Input: part model. Units: mm. Frame: model coordinates. Round coordinates to 2 decimals unless told otherwise and drop trailing zeros. Write each loop counter-clockwise with the first axis right and the second up, starting at its lowest first coordinate (ties: lowest second). Pieces come first, ordered by that corner, then holes. Notation, with made-up numbers: (47, -37) -> (51, -37) arc R32 cw to (51, -3) -> close; hole circle Ø2 at (21.5, 70.25). An arc over 180 degrees is marked (long way). Use CSV: the item, a comma, the result in double quotes.
Autodesk Inventor part; units mm, degrees
ref_plane "YZ Plane" through (0, 0, 0) normal (1, 0, 0) x (0, 1, 0)
ref_plane "XZ Plane" through (0, 0, 0) normal (0, 1, 0) x (-1, 0, 0)
ref_plane "XY Plane" through (0, 0, 0) normal (0, 0, 1) x (1, 0, 0)
sketch "Sketch1" plane through (0, 0, 0) normal (0, 1, 0) x (-1, 0, 0)
  line L0 (16.1925, 35.7868) -> (-9.2075, 35.7868)
  line L1 (-9.2075, 35.7868) -> (-9.2075, 10.3868)
  line L2 (-9.2075, 10.3868) -> (16.1925, 10.3868)
  line L3 (16.1925, 10.3868) -> (16.1925, 35.7868)
  point P0 (0, 0)
  dimension "d0" = 25.4
  dimension "d1" = 25.4
extrude "Extrusion1" add sketch "Sketch1" along normal blind 368.3
sketch "Sketch2" plane through (0, 368.3, 0) normal (0, 1, 0) x (1, 0, 0)
  line L0 (-9.8425, -16.7368) -> (2.8575, -16.7368)
  line L1 (2.8575, -16.7368) -> (2.8575, -1.003)
  line L2 (2.8575, -1.003) -> (-9.8425, -1.003)
  line L3 (-9.8425, -1.003) -> (-9.8425, -16.7368)
  line L4 (9.2075, -35.7868) -> (9.2075, -10.3868)
  line L5 (-16.1925, -10.3868) -> (-16.1925, -35.7868)
  line L6 (9.2075, -10.3868) -> (-16.1925, -10.3868)
  point P0 (0, 0)
  dimension "d4" = 6.35
  dimension "d5" = 6.35
  dimension "d6" = 6.35
extrude "Extrusion2" cut sketch "Sketch2" against normal blind 508
sketch "Sketch4" plane through (0, 368.3, 0) normal (0, 1, 0) x (1, 0, 0)
  line L0 (-9.8425, -29.4368) -> (2.8575, -29.4368)
  line L1 (2.8575, -29.4368) -> (2.8575, -45.8861)
  line L2 (2.8575, -45.8861) -> (-9.8425, -45.8861)
  line L3 (-9.8425, -45.8861) -> (-9.8425, -29.4368)
  line L4 (-16.1925, -10.3868) -> (-16.1925, -35.7868)
  line L5 (9.2075, -35.7868) -> (9.2075, -10.3868)
  line L6 (-16.1925, -35.7868) -> (9.2075, -35.7868)
  point P0 (0, 0)
  dimension "d20" = 6.35
  dimension "d21" = 6.35
  dimension "d22" = 6.35
extrude "Extrusion3" cut sketch "Sketch4" against normal blind 508
sketch "Sketch5" plane through (9.2075, 0, 10.3868) normal (0, 0, -1) x (-1, 0, 0)
  line L0 (0, 0) -> (6.35, 0)
  line L1 (0, 0) -> (0, 368.3)
  line L2 (25.4, 0) -> (25.4, 368.3)
  line L3 (19.05, 0) -> (25.4, 0)
  point P0 (9.2075, 0)
  point P1 (19.05, 6.35)
  point P2 (6.35, 12.7)
  dimension "d25" = 12.7
  dimension "d27" = 6.35
  dimension "d28" = 6.35
  dimension "d60" = 19.05
hole "Hole2" at (-9.8425, 6.35, 10.3868) at (2.8575, 12.7, 10.3868) direction (0, 0, 1) diameter 3.175 end through all
sketch "Sketch6" plane through (-16.1925, 0, 10.3868) normal (0, 0, -1) x (-1, 0, 0)
  line L0 (-6.35, 368.3) -> (-6.35, 7.9375)
  line L1 (-25.4, 368.3) -> (-19.05, 368.3)
  line L2 (-25.4, 0) -> (-25.4, 368.3)
  line L3 (-6.35, 368.3) -> (0, 368.3)
  line L4 (0, 0) -> (0, 368.3)
  point P0 (-16.1925, 0)
  point P1 (-19.05, 361.95)
  point P2 (-6.35, 355.6)
  dimension "d36" = 6.35
  dimension "d38" = 12.7
  dimension "d58" = 6.35
  dimension "d59" = 19.05
hole "Hole3" at (2.8575, 361.95, 10.3868) at (-9.8425, 355.6, 10.3868) direction (0, 0, 1) diameter 3.175 end through all
sketch "Sketch7" plane through (0, 0, 0) normal (0, -1, 0) x (1, 0, 0)
  line L0 (2.8575, 35.7868) -> (9.2075, 35.7868)
  line L1 (9.2075, 35.7868) -> (9.2075, 10.3868)
  line L2 (-16.1925, 10.3868) -> (-16.1925, 35.7868)
  line L3 (-16.1925, 35.7868) -> (-9.8425, 35.7868)
  point P0 (0, 0)
  point P1 (-9.8425, 23.0868)
  point P2 (2.8575, 23.0868)
  dimension "d47" = 12.7
  dimension "d48" = 6.35
  dimension "d49" = 6.35
  dimension "d50" = 12.7
hole "Hole4" at (-9.8425, 0, 23.0868) at (2.8575, 0, 23.0868) direction (0, 1, 0) diameter 3.175 end through all
properties part number "LeftSideElevator"
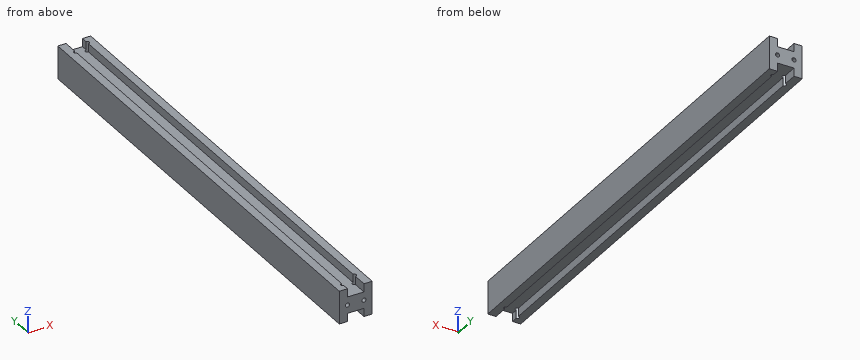
Item 1: Line query: line 1 (X direction, y = 206, z = 23.5); line 2 (Y direction, x = -10.25, z = 20.5); line 3 (Y direction, x = -10, z = 15.5). Output: solid intervals per line, ascending.
Worked answers:
line 1,"x = -16.19 to -11.38, -8.31 to 1.32, 4.39 to 9.21"
line 2,"y = 0 to 4.82, 7.88 to 354.07, 357.13 to 368.3"
line 3,"y = 0 to 4.77, 7.93 to 354.02, 357.18 to 368.3"
Item 2: Section query A-A on y = 249.5. Return the cut outline in (x, z) (1 decimal).
Worked answers:
outline,"(-16.2, 10.4) -> (-9.8, 10.4) -> (-9.8, 16.7) -> (2.9, 16.7) -> (2.9, 10.4) -> (9.2, 10.4) -> (9.2, 35.8) -> (2.9, 35.8) -> (2.9, 29.4) -> (-9.8, 29.4) -> (-9.8, 35.8) -> (-16.2, 35.8) -> close; hole circle Ø3.2 at (-9.8, 23.1); hole circle Ø3.2 at (2.9, 23.1)"
Item 3: First-contact query: pin 1 Ø3 at (x, y) = (-2.5, 279) entering from +Z; pin 2 Ø10 at (x, y) = (-3.5, 242) entering from -Z. Flat tips, straight axial feed; report the tip coordinate or a pass-through.
Worked answers:
pin 1,"stops at z = 29.44"
pin 2,"stops at z = 16.74"
